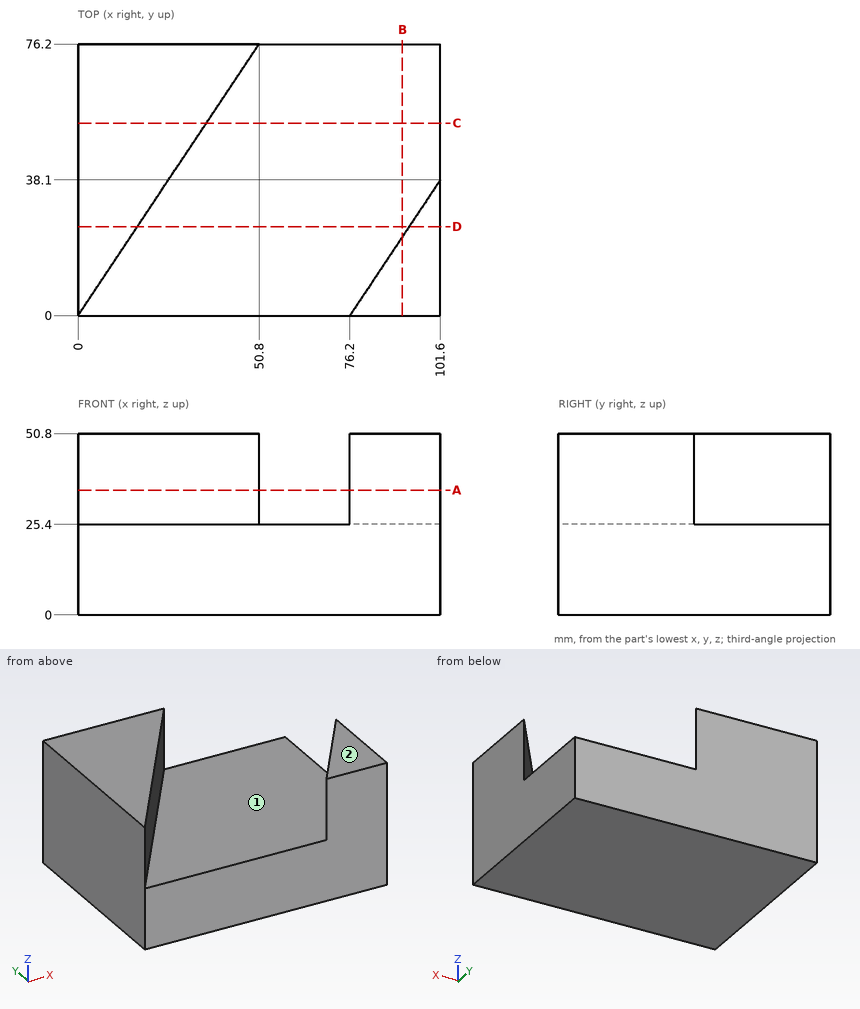
For this review, use the dimensioned drawing (mm, ordinates from the lowest corner) and the shaded views. A direction names the side the tool comes from. Give positions to 0.01 mm unless a question says otherwise; leave off trailing zeros. Write each loop counter-clockwise with the first axis right and the second up, starting at its lowest first coordinate (ties: lowest second). Pieces come first, ordered by that corner, then holes. Notation, with made-up numbers: M -19,-35 L 35,-35 A12 ccw 35,-17 Z; hole C 82.25,68.5 d6. An arc over 180 degrees is marked long. Write item = value, one per line. Start each with the question number.
Q1. We need section D-D (y = 25). State the section outline as (x, z) points, plus the area to 3 significant figures.
Q2. We need section B-B (x = 91). State the section outline as (y, z) points, plus the area to 3 significant figures.
Q3. Machinability: for the marked faces 1 and 2, which of the approach directions +Z, -Z, +X, -X, +Y, -Y give a long, thin tool a straight path to every point of the face, cutting with its end or side? Answer none if there is none.
Q4. For line 1 (Z direction, x = 83.5, y = 59); line 2 (X direction, y = 22.5, z = 34.5); line 3 (X direction, y = 11, z = 26), list the stretches that pass through material, from the lowest coordinate up.
Q5. We need section C-C (y = 54). State the section outline as (x, z) points, plus the area to 3 significant figures.
Q6. Clearance check with a flat-ended pin moving along its axis: pin 1 (3 mm diameter, centred on y = 55.5, z = 34.5, fed in from +X). State where the tip first meets the part, or that it passes through.
Q7. We need section A-A (z = 35). State the section outline as (x, y) points, plus the area to 3 significant figures.
Result set:
q1.outline = M 0,0 L 101.6,0 L 101.6,50.8 L 92.87,50.8 L 92.87,25.4 L 16.67,25.4 L 16.67,50.8 L 0,50.8 Z
q1.area = 3,230 mm2
q2.outline = M 0,0 L 76.2,0 L 76.2,25.4 L 22.2,25.4 L 22.2,50.8 L 0,50.8 Z
q2.area = 2,500 mm2
q3.face_1 = +Z
q3.face_2 = +Z, +X, -X, +Y, -Y
q4.line_1 = 0 to 25.4
q4.line_2 = 0 to 15, 91.2 to 101.6
q4.line_3 = 0 to 7.33, 83.53 to 101.6
q5.outline = M 0,0 L 101.6,0 L 101.6,25.4 L 36,25.4 L 36,50.8 L 0,50.8 Z
q5.area = 3,500 mm2
q6.pin_1 = 38
q7.outline = M 0,0 L 50.8,76.2 L 0,76.2 Z; M 76.2,0 L 101.6,0 L 101.6,38.1 Z
q7.area = 2,420 mm2
